Part model, mm, in its own coordinate system. Coordinates: 2 decimals unless noted, no trailing zeros. Write each loop counter-clockwise with the first axis right and the second up, starting at its lowest first coordinate (ties: lowest second). Pieces come first, ordered by that corner, then holes. Notation, with made-up numbers: (31, 33.25) -> (89, 33.25) arc R23 cw to (89, 54.25) -> close; hole circle Ø11 at (77, -40). An arc over 180 degrees is marked (long way). Write item = value, one per line. Start each with the question number.
Q1. Pin check, flat tips, straight feed: P1, Ø3, axis at x = -7.5, y = -10.5, coming from the +Z side; P2, Ø4, axis at x = -37.74, y = -12.74, coming from the -Z side (3 decimals). Stop position of each tip, or through.
Q2. Band-saw the part on D-D, the plane y = 12. List the corners of the cut face in (x, z).
Q3. Band-saw the part on C-C, the plane z = -0.85. Give the number of separate pieces and of enclosed holes in the cut face, plus the area to 3 significant figures.
Q4. Band-saw the part on A-A, the plane x = 0. List the corners of the cut face in (y, z), plus the area to 3 significant figures.
Q5. Probe line 1 (X direction, y = 0, z = -3.95); line 2 (X direction, y = -11, z = -2.35); line 3 (X direction, y = 2.5, z = -4.35). List the from-to ranges inside material, lowest first.
Q6. Band-saw the part on B-B, the plane y = 0. List the corners of the cut face in (x, z), plus the area to 3 significant figures.
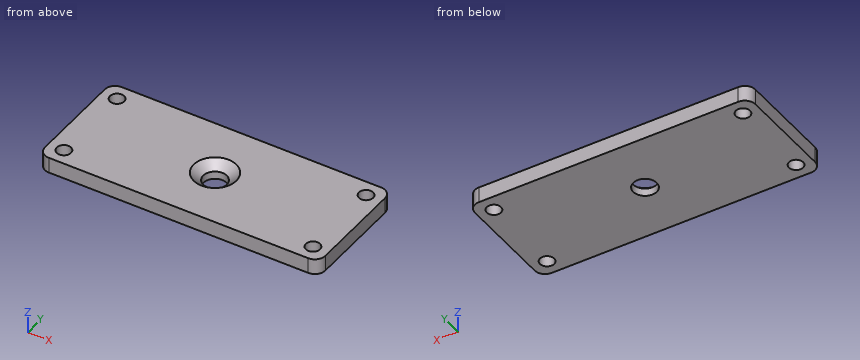
from build123d import *

# Parameters (mm, degrees)
SKETCH1_W           = 85
SKETCH1_H           = 4.7625
BOSS_EXTRUDE1_DEPTH = 17.5
FILLET1_R           = 3.175
SKETCH3_R           = 2.159
CUT_EXTRUDE3_DEPTH  = 10


with BuildPart() as part:
    # Sketch1 → Boss-Extrude1 (new, symmetric)
    with BuildSketch(Plane(origin=(0, 0, 0), x_dir=(1, 0, 0), z_dir=(0, 1, 0))):
        with Locations((0, 2.38125)):
            Rectangle(SKETCH1_W, SKETCH1_H)
    extrude(amount=BOSS_EXTRUDE1_DEPTH, both=True)

    # Fillet1
    fillet1_edges = [part.edges().sort_by_distance(p)[0] for p in [
        (42.5, 17.5, -2.38125),
        (42.5, -17.5, -2.38125),
        (-42.5, -17.5, -2.38125),
        (-42.5, 17.5, -2.38125),
    ]]
    fillet(fillet1_edges, radius=FILLET1_R)

    # Sketch3 → Cut-Extrude3 (cut)
    with BuildSketch(Plane.XY):
        with Locations((-37.7375, 12.7375)):
            Circle(SKETCH3_R)
        with Locations((-37.7375, -12.7375)):
            Circle(SKETCH3_R)
        with Locations((37.7375, 12.7375)):
            Circle(SKETCH3_R)
        with Locations((37.7375, -12.7375)):
            Circle(SKETCH3_R)
    extrude(amount=-CUT_EXTRUDE3_DEPTH, mode=Mode.SUBTRACT)

    # Sketch9 → CSK for 1/4 Flat Head Machine Screw (100)1 (revolve, cut)
    with BuildSketch(Plane(origin=(0, 0, 0), x_dir=(0, -1, 0), z_dir=(1, 0, 0))):
        Polygon((0, 0), (0, 4.7625), (3.57124, 4.7625), (3.57124, 2.406252448), (6.4389, 0), align=None)
    revolve(axis=Axis((0, 0, 6.35), (0, 0, -1)), mode=Mode.SUBTRACT)


solid = part.part
Ans:
q1.P1 = 0
q1.P2 = through
q2.outline = (-42.5, -4.76) -> (-39.77, -4.76) -> (-39.77, 0) -> (-42.5, 0) -> close; (-35.71, -4.76) -> (35.71, -4.76) -> (35.71, 0) -> (-35.71, 0) -> close; (39.77, -4.76) -> (42.5, -4.76) -> (42.5, 0) -> (39.77, 0) -> close
q3.separate_pieces = 1
q3.enclosed_holes = 5
q3.area = 2,820 mm2
q4.outline = (-17.5, -4.76) -> (-3.57, -4.76) -> (-3.57, -2.41) -> (-6.44, 0) -> (-17.5, 0) -> close; (3.57, -4.76) -> (17.5, -4.76) -> (17.5, 0) -> (6.44, 0) -> (3.57, -2.41) -> close
q4.area = 126 mm2
q5.line_1 = -42.5 to -3.57, 3.57 to 42.5
q5.line_2 = -42.5 to -39.02, -36.46 to 36.46, 39.02 to 42.5
q5.line_3 = -42.5 to -2.55, 2.55 to 42.5
q6.outline = (-42.5, -4.76) -> (-3.57, -4.76) -> (-3.57, -2.41) -> (-6.44, 0) -> (-42.5, 0) -> close; (3.57, -4.76) -> (42.5, -4.76) -> (42.5, 0) -> (6.44, 0) -> (3.57, -2.41) -> close
q6.area = 364 mm2
